For this review, take the finished solid that the model builds, in its own axes (mm). Round coordinates to 2 decimals unless told otherwise and drop trailing zeros. Write each loop counter-clockwise with the first axis right and the second up, starting at its lowest first coordinate (ties: lowest second). Pieces come first, ordered by that corner, then holes. Notation, with made-up numbers: (37.5, 27.25) -> (86.5, 27.25) arc R20 ccw to (86.5, 56.25) -> close; hole circle Ø7 at (-0.5, -26.75). An arc over 180 degrees is marked (long way). Answer in a Markdown table with one row per item. Add a question column.
```python
from build123d import *

# Parameters (mm, degrees)
F0_W         = 113.590836525
F0_H         = 63.365586102
F0_R         = 13.6776668511
F0_R_2       = 12.9483089266
F0_R_3       = 13.3718975465
F0_R_4       = 13.6714310258
F0_R_5       = 14.0406678545
F0_R_6       = 13.4346835475
F1_DEPTH     = 25.4
F2_W         = 109.635181725
F2_H         = 62.0416179299
F2_R         = 13.6776668511
F2_R_2       = 12.9483089266
F2_R_3       = 13.3718975465
F2_R_4       = 13.6714310258
F2_R_5       = 14.0406678545
F2_R_6       = 13.4346835475
F3_DEPTH     = 12.7
F4_T1_DEPTH  = 6.4524666085
F4_T3_DEPTH  = 6.4524666085
F4_T5_DEPTH  = 6.4524666085
F4_T7_DEPTH  = 6.4524666085
F4_T9_DEPTH  = 6.4524666085
F4_T11_DEPTH = 6.4524666085
F4_T13_DEPTH = 6.4524666085
F4_T15_DEPTH = 6.4524666085
F4_T17_DEPTH = 89.4938852597
F4_T19_DEPTH = 139.7191356827
F4_T21_DEPTH = 51.5282991577


# Not quite as in the source:
# - a fillet or chamfer that OpenCascade refuses, or shapes differently, is made with other operations: its cross-section is extruded or revolved along the edge and cut away or added


with BuildPart() as f1:
    # F0 (on Top) → F1 (new body)
    with BuildSketch(Plane.XY):
        Rectangle(F0_W, F0_H)
        with Locations((-35.1868793368, -16.4984129369)):
            Circle(F0_R, mode=Mode.SUBTRACT)
        with Locations((0, -16.790419817)):
            Circle(F0_R_2, mode=Mode.SUBTRACT)
        with Locations((37.5229418278, -16.4984129369)):
            Circle(F0_R_3, mode=Mode.SUBTRACT)
        with Locations((-34.0188518167, 16.2064060569)):
            Circle(F0_R_4, mode=Mode.SUBTRACT)
        with Locations((37.2309349477, 15.6223904341)):
            Circle(F0_R_5, mode=Mode.SUBTRACT)
        with Locations((0, 16.4984129369)):
            Circle(F0_R_6, mode=Mode.SUBTRACT)
    extrude(amount=F1_DEPTH)

    # F2 (on face) → F3 (join)
    with BuildSketch(Plane.XY):
        Rectangle(F2_W, F2_H)
        with Locations((-35.1868793368, -16.4984129369)):
            Circle(F2_R, mode=Mode.SUBTRACT)
        with Locations((0, -16.790419817)):
            Circle(F2_R_2, mode=Mode.SUBTRACT)
        with Locations((37.5229418278, -16.4984129369)):
            Circle(F2_R_3, mode=Mode.SUBTRACT)
        with Locations((-34.0188518167, 16.2064060569)):
            Circle(F2_R_4, mode=Mode.SUBTRACT)
        with Locations((37.2309349477, 15.6223904341)):
            Circle(F2_R_5, mode=Mode.SUBTRACT)
        with Locations((0, 16.4984129369)):
            Circle(F2_R_6, mode=Mode.SUBTRACT)
    extrude(amount=F3_DEPTH)

    # F4: chamfer of 5.08 on 12 edges, made by hand

    # F4_s2 → F4_t1 (cut)
    with BuildSketch(Plane(origin=(26.1060704378, -26.1060704378, -26.1060704378), x_dir=(0.7071067812, 0.7071067812, 0), z_dir=(0.5773502692, -0.5773502692, -0.5773502692))):
        Polygon((14.165205132, 38.1949798276), (17.7573075804, 31.9732758809), (21.3494100289, 38.1949798276), align=None)
    extrude(amount=F4_T1_DEPTH, mode=Mode.SUBTRACT)

    # F4_s4 → F4_t3 (cut)
    with BuildSketch(Plane(origin=(26.1060704378, 26.1060704378, -26.1060704378), x_dir=(-0.7071067812, 0.7071067812, 0), z_dir=(0.5773502692, 0.5773502692, -0.5773502692))):
        Polygon((-14.165205132, 38.1949798276), (-17.7573075804, 31.9732758809), (-21.3494100289, 38.1949798276), align=None)
    extrude(amount=F4_T3_DEPTH, mode=Mode.SUBTRACT)

    # F4_s6 → F4_t5 (cut)
    with BuildSketch(Plane(origin=(-26.1060704378, 26.1060704378, -26.1060704378), x_dir=(-0.7071067812, -0.7071067812, 0), z_dir=(-0.5773502692, 0.5773502692, -0.5773502692))):
        Polygon((14.165205132, 38.1949798276), (17.7573075804, 31.9732758809), (21.3494100289, 38.1949798276), align=None)
    extrude(amount=F4_T5_DEPTH, mode=Mode.SUBTRACT)

    # F4_s8 → F4_t7 (cut)
    with BuildSketch(Plane(origin=(-26.1060704378, -26.1060704378, -26.1060704378), x_dir=(0.7071067812, -0.7071067812, 0), z_dir=(-0.5773502692, -0.5773502692, -0.5773502692))):
        Polygon((-14.165205132, 38.1949798276), (-17.7573075804, 31.9732758809), (-21.3494100289, 38.1949798276), align=None)
    extrude(amount=F4_T7_DEPTH, mode=Mode.SUBTRACT)

    # F4_s10 → F4_t9 (cut)
    with BuildSketch(Plane(origin=(-34.5727371045, 34.5727371045, 34.5727371045), x_dir=(-0.7071067812, -0.7071067812, 0), z_dir=(-0.5773502692, 0.5773502692, 0.5773502692))):
        Polygon((14.165205132, -17.455966672), (17.7573075804, -11.2342627254), (21.3494100289, -17.455966672), align=None)
    extrude(amount=F4_T9_DEPTH, mode=Mode.SUBTRACT)

    # F4_s12 → F4_t11 (cut)
    with BuildSketch(Plane(origin=(34.5727371045, -34.5727371045, 34.5727371045), x_dir=(0.7071067812, 0.7071067812, 0), z_dir=(0.5773502692, -0.5773502692, 0.5773502692))):
        Polygon((14.165205132, -17.455966672), (17.7573075804, -11.2342627254), (21.3494100289, -17.455966672), align=None)
    extrude(amount=F4_T11_DEPTH, mode=Mode.SUBTRACT)

    # F4_s14 → F4_t13 (cut)
    with BuildSketch(Plane(origin=(34.5727371045, 34.5727371045, 34.5727371045), x_dir=(-0.7071067812, 0.7071067812, 0), z_dir=(0.5773502692, 0.5773502692, 0.5773502692))):
        Polygon((-14.165205132, -17.455966672), (-17.7573075804, -11.2342627254), (-21.3494100289, -17.455966672), align=None)
    extrude(amount=F4_T13_DEPTH, mode=Mode.SUBTRACT)

    # F4_s16 → F4_t15 (cut)
    with BuildSketch(Plane(origin=(-34.5727371045, -34.5727371045, 34.5727371045), x_dir=(0.7071067812, -0.7071067812, 0), z_dir=(-0.5773502692, -0.5773502692, 0.5773502692))):
        Polygon((-14.165205132, -17.455966672), (-17.7573075804, -11.2342627254), (-21.3494100289, -17.455966672), align=None)
    extrude(amount=F4_T15_DEPTH, mode=Mode.SUBTRACT)

    # F4_s18 → F4_t17 (cut)
    with BuildSketch(Plane.XZ.offset(-44.7469426299)):
        Polygon((51.7154182625, 0), (56.7954182625, 5.08), (56.7954182625, 0), align=None)
        Polygon((-51.7154182625, 0), (-56.7954182625, 5.08), (-56.7954182625, 0), align=None)
        Polygon((-51.7154182625, 25.4), (-56.7954182625, 20.32), (-56.7954182625, 25.4), align=None)
        Polygon((51.7154182625, 25.4), (56.7954182625, 20.32), (56.7954182625, 25.4), align=None)
    extrude(amount=F4_T17_DEPTH, mode=Mode.SUBTRACT)

    # F4_s20 → F4_t19 (cut)
    with BuildSketch(Plane.YZ.offset(-69.8595678413)):
        Polygon((31.682793051, 5.08), (26.602793051, 0), (31.682793051, 0), align=None)
        Polygon((-31.682793051, 5.08), (-26.602793051, 0), (-31.682793051, 0), align=None)
        Polygon((31.682793051, 20.32), (26.602793051, 25.4), (31.682793051, 25.4), align=None)
        Polygon((-26.602793051, 25.4), (-31.682793051, 20.32), (-31.682793051, 25.4), align=None)
    extrude(amount=F4_T19_DEPTH, mode=Mode.SUBTRACT)

    # F4_s22 → F4_t21 (cut)
    with BuildSketch(Plane.XY.offset(-13.0641495789)):
        Polygon((-51.7154182625, 31.682793051), (-56.7954182625, 26.602793051), (-56.7954182625, 31.682793051), align=None)
        Polygon((51.7154182625, -31.682793051), (56.7954182625, -26.602793051), (56.7954182625, -31.682793051), align=None)
        Polygon((-51.7154182625, -31.682793051), (-56.7954182625, -26.602793051), (-56.7954182625, -31.682793051), align=None)
        Polygon((51.7154182625, 31.682793051), (56.7954182625, 26.602793051), (56.7954182625, 31.682793051), align=None)
    extrude(amount=F4_T21_DEPTH, mode=Mode.SUBTRACT)


solid = f1.part
```
1. We need section D-D (y = -1.5). Write out the cut boundary in (x, z).
2. For L1, parallel to Y at x = 0, z = 11.5; L2, parallel to X at y = 12.5, z = 11; L3, parallel to Y at x = -3, z = 9.75, list the stretches that pass through material, from the lowest coordinate up. Write a range as [from, to].
3. The part is to be moulded in two halves that separate along Y. For faces 1 (the flat face through (53.25, 28.21, 3.14)), 2 (the cylindrical face through (35.78, -3.24, 12.52)), 3 (the cylindrical face through (-1.686, -3.952, 12.522)), 4 (the flat face through (-1, -31.683, 13)), say which applies: pulls with the +Y half, pulls with the -Y half, needs draft (parallel to the pull), parting line crosses it, or undercut.
4. We need section A-A (x = 18). Write out the cut boundary in (y, z).
5. We need section B-B (y = 7). Write out the cut boundary in (x, z).
6. We need section C-C (z = 17). Write out the cut boundary in (x, y), plus the area to 3 significant figures.
Response:
| question | item | result |
|---|---|---|
| 1 | outline | (-56.8, 5.08) -> (-51.72, 0) -> (51.72, 0) -> (56.8, 5.08) -> (56.8, 20.32) -> (51.72, 25.4) -> (-51.72, 25.4) -> (-56.8, 20.32) -> close |
| 2 | L1 | [-31.68, -29.74], [-3.84, 3.06], [29.93, 31.68] |
| 2 | L2 | [-56.8, -47.18], [-20.86, -12.83], [12.83, 23.54], [50.92, 56.8] |
| 2 | L3 | [-31.68, -29.39], [-4.19, 3.4], [29.59, 31.68] |
| 3 | face 1 | pulls with the +Y half |
| 3 | face 2 | undercut |
| 3 | face 3 | undercut |
| 3 | face 4 | pulls with the -Y half |
| 4 | outline | (-31.68, 5.08) -> (-26.6, 0) -> (26.6, 0) -> (31.68, 5.08) -> (31.68, 20.32) -> (26.6, 25.4) -> (-26.6, 25.4) -> (-31.68, 20.32) -> close |
| 5 | outline | (-56.8, 5.08) -> (-51.72, 0) -> (-44.13, 0) -> (-44.13, 25.4) -> (-51.72, 25.4) -> (-56.8, 20.32) -> close; (-23.91, 0) -> (-9.5, 0) -> (-9.5, 25.4) -> (-23.91, 25.4) -> close; (9.5, 0) -> (26.15, 0) -> (26.15, 25.4) -> (9.5, 25.4) -> close; (48.31, 0) -> (51.72, 0) -> (56.8, 5.08) -> (56.8, 20.32) -> (51.72, 25.4) -> (48.31, 25.4) -> close |
| 6 | outline | (-56.8, -26.6) -> (-51.72, -31.68) -> (51.72, -31.68) -> (56.8, -26.6) -> (56.8, 26.6) -> (51.72, 31.68) -> (-51.72, 31.68) -> (-56.8, 26.6) -> close; hole circle Ø27.36 at (-35.19, -16.5); hole circle Ø27.34 at (-34.02, 16.21); hole circle Ø26.87 at (0, 16.5); hole circle Ø25.9 at (0, -16.79); hole circle Ø28.08 at (37.23, 15.62); hole circle Ø26.74 at (37.52, -16.5) |
| 6 | area | 3,700 mm2 |
